Verification items for the finished model (mm, model axes). Face numbers are marked on the shaded views. A direction names the side the tool comes from. Coordinates: 2 decimals unless noted, no trailing zeros. Order: outer loops, then holes, each group sorted by start corner. A loop starts at its lowest first (then second) coordinate and runs counter-clockwise, first axis right, second up. Notation, with made-up numbers: M 5.5,40.5 L 13.5,40.5 A31 cw 13.5,77.5 Z; hole C 37,34 d4. An arc over 180 degrees is marked long. Return JSON: item names as keys, results as strings.
```python
from build123d import *

# Parameters (mm, degrees)
BOSS_EXTRUDE1_DEPTH              = 4.7625
F_6_CLEARANCE_HOLE1_D            = 4.3053
F_3_4_0_75_DIAMETER_HOLE1_D      = 19.05
F_13_32_0_40625_DIAMETER_HOLE1_D = 10.31875


with BuildPart() as part:
    # Sketch1 → Boss-Extrude1 (new body)
    with BuildSketch(Plane.XY):
        with BuildLine():
            Line((-17.78404549, -88.20554549), (-0.69445451, -71.11595451))
            ThreePointArc((-0.69445451, -71.11595451), (-0.474213395, -70.786340388), (-0.396875, -70.397534021))
            Line((-0.396875, -70.397534021), (-0.396875, -12.92225))
            ThreePointArc((-0.396875, -12.92225), (-0.69445451, -12.20382951), (-1.412875, -11.90625))
            Line((-1.412875, -11.90625), (-7.14375, -11.90625))
            ThreePointArc((-7.14375, -11.90625), (-10.511346045, -10.511346045), (-11.90625, -7.14375))
            Line((-11.90625, -7.14375), (-11.90625, -1.412875))
            ThreePointArc((-11.90625, -1.412875), (-12.20382951, -0.69445451), (-12.92225, -0.396875))
            Line((-12.92225, -0.396875), (-33.0835, -0.396875))
            ThreePointArc((-33.0835, -0.396875), (-33.80192049, -0.69445451), (-34.0995, -1.412875))
            Line((-34.0995, -1.412875), (-34.0995, -15.131583582))
            ThreePointArc((-34.0995, -15.131583582), (-34.01851745, -15.529073666), (-33.788479592, -15.863198081))
            ThreePointArc((-33.788479592, -15.863198081), (-29.070029057, -33.446687471), (-42.397902867, -45.848729815))
            add(Edge.make_bspline(
                [(-42.397902867, -45.848729815), (-45.551783199, -47.860753205), (-48.991026243, -46.228)],
                knots=[-2.210610991, -2.210610991, -2.210610991, -1.065002144, -1.065002144, -1.065002144], degree=2, weights=[1, 0.84038431, 1]))
            Line((-48.991026243, -46.228), (-63.674625, -46.228))
            ThreePointArc((-63.674625, -46.228), (-64.39304549, -46.52557951), (-64.690625, -47.244))
            Line((-64.690625, -47.244), (-64.690625, -75.97775))
            ThreePointArc((-64.690625, -75.97775), (-64.39304549, -76.69617049), (-63.674625, -76.99375))
            Line((-63.674625, -76.99375), (-57.94375, -76.99375))
            ThreePointArc((-57.94375, -76.99375), (-54.576153955, -78.388653955), (-53.18125, -81.75625))
            Line((-53.18125, -81.75625), (-53.18125, -87.487125))
            ThreePointArc((-53.18125, -87.487125), (-52.88367049, -88.20554549), (-52.16525, -88.503125))
            Line((-52.16525, -88.503125), (-18.502465979, -88.503125))
            ThreePointArc((-18.502465979, -88.503125), (-18.113659612, -88.425786605), (-17.78404549, -88.20554549))
        make_face()
    extrude(amount=BOSS_EXTRUDE1_DEPTH)

    # #6 Clearance Hole1 (through all)
    with Locations(Plane.XY.offset(4.7625)):
        with Locations((-57.15, -67.31), (-23.1775, -12.7)):
            Hole(F_6_CLEARANCE_HOLE1_D / 2)

    # 3/4 (0.75) Diameter Hole1 (through all)
    with Locations(Plane.XY.offset(4.7625)):
        with Locations((-16.8275, -27.94)):
            Hole(F_3_4_0_75_DIAMETER_HOLE1_D / 2)

    # 13/32 (0.40625) Diameter Hole1 (through all)
    with Locations(Plane.XY.offset(4.7625)):
        with Locations((-9.2075, -65.0875)):
            Hole(F_13_32_0_40625_DIAMETER_HOLE1_D / 2)


solid = part.part
```
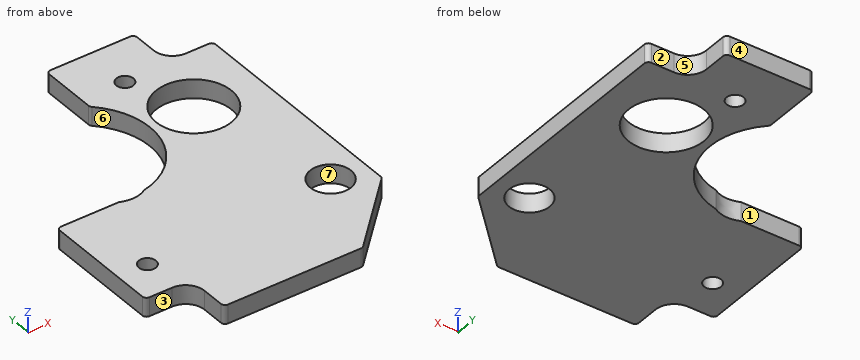
Q1. Draft check along X on the marked faces 4, 5, 6 and 7. Enter one of: pulls with the +X half, pulls with the -X half, needs draft (parallel to the pull), parting line crosses it, or undercut.
Values:
{"face 4": "needs draft", "face 5": "pulls with the +X half", "face 6": "pulls with the -X half", "face 7": "undercut"}
Q2. Tool access check on the marked faces 1, 2 and 3. Record the directions out of +Z, -Z, +X, -X, +Y, -Y that give a thin tool (end or side, any length) a straight path to the whole face; none if there is none.
Values:
{"face 1": "+Z, -Z, -X, +Y", "face 2": "+Z, -Z, +X, +Y", "face 3": "+Z, -Z, -X, -Y"}
Q3. Cross-section at D-D, the plane y = -39.5. Record the boundary of the cut face in (x, z), and give its area (3 significant figures).
Values:
{"outline": "M -32.17,0 L -0.4,0 L -0.4,4.76 L -32.17,4.76 Z", "area": "151 mm^2"}
Q4. Cross-section at B-B, the plane x = -23. Record the boundary of the cut face in (y, z).
Values:
{"outline": "M -88.5,0 L -35.19,0 L -35.19,4.76 L -88.5,4.76 Z; M -20.69,0 L -14.85,0 L -14.85,4.76 L -20.69,4.76 Z; M -10.55,0 L -0.4,0 L -0.4,4.76 L -10.55,4.76 Z"}
Q5. Cross-section at C-C, the plane z = 3.8. State how many separate pieces and enclosed holes the cut face has, and give its area (3 significant figures).
Values:
{"separate pieces": "1", "enclosed holes": "4", "area": "3,360 mm^2"}
Q6. Go/stop test with flat-tipped pins: pin 1 (1.4 mm diameter, centred on x = -61.5, z = 3, fed in from -Y); pin 2 (2.5 mm diameter, centred on y = -4, z = 2, fed in from +X); pin 3 (1 mm diameter, centred on x = -46.5, z = 4, fed in from +Y). Record where each tip stops, or that it passes through.
Values:
{"pin 1": "y = -76.99", "pin 2": "x = -11.91", "pin 3": "y = -46.82"}
Q7. Cross-section at A-A, the plane y = -62.5. Record the boundary of the cut face in (x, z).
Values:
{"outline": "M -64.69,0 L -13.67,0 L -13.67,4.76 L -64.69,4.76 Z; M -4.74,0 L -0.4,0 L -0.4,4.76 L -4.74,4.76 Z"}
Q8. Material ranges on line 1 along X through (y, z) = (-68, 0.35); line 2 along Y through (x, z) = (-24, 3.75); line 3 along Y through (x, z) = (-58, 2.25), recorded low to high.
Values:
{"line 1": "-64.69 to -59.19, -55.11 to -13.47, -4.95 to -0.4", "line 2": "-88.5 to -34.21, -21.67 to -14.69, -10.71 to -0.4", "line 3": "-76.99 to -69.29, -65.33 to -46.23"}
